```python
from build123d import *

# Parameters (mm, degrees)
SKETCH3_R               = 28
BOSS_EXTRUDE1_DEPTH     = 5.15
SKETCH6_R               = 25
BOSS_EXTRUDE4_DEPTH     = 7
SKETCH7_R               = 3.4
BOSS_EXTRUDE5_DEPTH     = 10
CUT_EXTRUDE1_DEPTH      = 10
CUT_EXTRUDE1_DEPTH_BACK = 43.3971992
SKETCH8_R               = 1.65
CUT_EXTRUDE3_DEPTH      = 2.7
CHAMFER1_SIZE           = 1


with BuildPart() as part:
    # Sketch3 → Boss-Extrude1 (new body)
    with BuildSketch(Plane(origin=(0, 0, 0), x_dir=(1, 0, 0), z_dir=(0, 1, 0))):
        with Locations(Location((0, 0, 0), (0, 0, 90))):
            Circle(SKETCH3_R)
    extrude(amount=BOSS_EXTRUDE1_DEPTH)

    # Sketch6 → Boss-Extrude4 (add)
    with BuildSketch(Plane.XZ):
        with Locations(Location((0, 0, 0), (0, 0, 270))):
            Circle(SKETCH6_R)
    extrude(amount=BOSS_EXTRUDE4_DEPTH)

    # Sketch7 → Boss-Extrude5 (add)
    with BuildSketch(Plane(origin=(0, 5.15, 0), x_dir=(1, 0, 0), z_dir=(0, 1, 0))):
        with Locations(Location((-0.954174099, -21.854179847, 0), (0, 0, 270))):
            Circle(SKETCH7_R)
        with Locations(Location((-18.449187877, 11.753428933, 0), (0, 0, 270))):
            Circle(SKETCH7_R)
        with Locations(Location((19.403361976, 10.100750915, 0), (0, 0, 270))):
            Circle(SKETCH7_R)
    extrude(amount=BOSS_EXTRUDE5_DEPTH)

    # Sketch8 → Cut-Extrude1 (cut, two sides: drawn at the far end of the back side and taken through both)
    with BuildSketch(Plane.XZ.offset(-CUT_EXTRUDE1_DEPTH_BACK)):
        with Locations(Location((20, 0, 0), (0, 0, 90))):
            Circle(SKETCH8_R)
        with Locations(Location((-20, 0, 0), (0, 0, 90))):
            Circle(SKETCH8_R)
        with Locations(Location((11.471528727, 16.383040886, 0), (0, 0, 90))):
            Circle(SKETCH8_R)
        with Locations(Location((-11.471528727, -16.383040886, 0), (0, 0, 90))):
            Circle(SKETCH8_R)
        with Locations(Location((11.471528727, -16.383040886, 0), (0, 0, 90))):
            Circle(SKETCH8_R)
        with Locations(Location((-11.471528727, 16.383040886, 0), (0, 0, 90))):
            Circle(SKETCH8_R)
    extrude(amount=CUT_EXTRUDE1_DEPTH + CUT_EXTRUDE1_DEPTH_BACK, mode=Mode.SUBTRACT)

    # Sketch11 → Cut-Extrude3 (cut)
    with BuildSketch(Plane(origin=(0, 5.15, 0), x_dir=(1, 0, 0), z_dir=(0, 1, 0))):
        Polygon((11.858091258, -19.360271603), (14.243167426, -17.536883273), (13.856604896, -14.559652555), (11.084966196, -13.405810169), (8.699890028, -15.229198499), (9.086452558, -18.206429216), align=None)
        Polygon((-12.091418901, -19.320568674), (-9.237500125, -18.388645418), (-8.617609951, -15.45111763), (-10.851638553, -13.445513098), (-13.705557329, -14.377436353), (-14.325447503, -17.314964141), align=None)
        Polygon((-22.590586111, -1.517299224), (-19.981273382, -3.002162995), (-17.390687271, -1.48486377), (-17.409413889, 1.517299224), (-20.018726618, 3.002162995), (-22.609312729, 1.48486377), align=None)
        Polygon((20, -3.0022214), (22.6, -1.5011107), (22.6, 1.5011107), (20, 3.0022214), (17.4, 1.5011107), (17.4, -1.5011107), align=None)
        Polygon((9.008253879, 14.666762832), (11.726231698, 13.391643264), (14.189506546, 15.107921318), (13.934803575, 18.09931894), (11.216825756, 19.374438507), (8.753550908, 17.658160453), align=None)
        Polygon((-10.729703857, 13.473912288), (-8.581237024, 15.57091577), (-9.323061894, 18.480044367), (-12.213353597, 19.292169483), (-14.36182043, 17.195166002), (-13.61999556, 14.286037405), align=None)
    extrude(amount=-CUT_EXTRUDE3_DEPTH, mode=Mode.SUBTRACT)

    # Chamfer1
    chamfer1_edges = [part.edges().sort_by_distance(p)[0] for p in [
        (-18.449187877, 5.15, -15.153428933),
        (-0.954174099, 5.15, 18.454179847),
        (19.403361976, 5.15, -13.500750915),
    ]]
    chamfer(chamfer1_edges, length=CHAMFER1_SIZE)


solid = part.part
```
Design review of the part built by this model. Coordinates are the model's own, in mm. A direction names the side the tool comes from. Give positions to 0.01 mm unless a question says otherwise; leave off trailing zeros. Loops run counter-clockwise (first coordinate to the right, second up) from the corner with the lowest first, then second, coordinate; pieces in that order, holes last. Notation, with made-up numbers: M 9.5,69 L 35.5,69 A24 cw 35.5,96 Z; hole C 28,47.5 d9. An arc over 180 degrees is marked long. Return JSON: item names as keys, results as strings. Group by question number.
Item 1: For probe 1 along X at (y, z) = (1.75, 17); probe 2 along X at (y, z) = (-0.5, -0.5) (3 decimals); probe 3 along Y at (x, z) = (15, 10), list the stretches that pass through material, from the lowest coordinate up.
Item 2: We need section B-B (y = -0.75). Give the boundary of the cut face in (x, z), and give its area (3 significant figures).
Item 3: We need section C-C (y = 7.75). Give the boundary of the cut face in (x, z).
Item 4: Insertion check: pin 1 Ø4.5 at (x, z) = (11.5, 15.5) entering from +Y; pin 2 Ø12 at (x, y) = (-20, -2.5) entering from -Z; pin 3 Ø4 at (x, z) = (11.47, 16.38) entering from +Y; pin 4 Ø2.5 at (x, z) = (11.47, -16.38) entering from -Y. Each pin has a flat end and moves straight along its axis. Give the tip position at first contact, or say it passes through.
Item 5: We need section A-A (z = 16.5). Give the boundary of the cut face in (x, y), and give its area (3 significant figures).
Item 6: Mouldability with a two-part tool opening along X and no side actions: class faces 3 (the flat face through (-10, 2.45, 18)), 4 (the flat face through (-1, 15.15, 22)) as released by +X, released by -X, zero draft, split by the parting line, or undercut.
Item 7: Tool access review of faces 1 (the flat face through (-12.259, 3.819, 13.905)), 2 (the cylindrical face through (12.103, -2.209, -14.859)): name each direction out of +Z, -Z, +X, -X, +Y, -Y from which nothing blocks a thin tool from reaching the whole face with its end or side.
Item 8: We need section D-D (z = -23). Give the boundary of the cut face in (x, y).
Output:
{
 "1": {"probe 1": "x = -22.25 to -13, -9.94 to 9.94, 13 to 22.25", "probe 2": "x = -24.995 to -21.572, -18.428 to 18.428, 21.572 to 24.995", "probe 3": "y = -7 to 5.15"},
 "2": {"outline": "C 0,0 d50; hole C -20,0 d3.3; hole C -11.47,-16.38 d3.3; hole C -11.47,16.38 d3.3; hole C 11.47,-16.38 d3.3; hole C 11.47,16.38 d3.3; hole C 20,0 d3.3", "area": "1,910 mm^2"},
 "3": {"outline": "C -18.45,-11.75 d6.8; C -0.95,21.85 d6.8; C 19.4,-10.1 d6.8"},
 "4": {"pin 1": "stops at y = 5.15", "pin 2": "stops at z = -23.93", "pin 3": "stops at y = 2.45", "pin 4": "passes through"},
 "5": {"outline": "M -22.62,0 L -18.78,0 L -18.78,-7 L -13.12,-7 L -13.12,2.45 L -14.15,2.45 L -14.15,5.15 L -22.62,5.15 Z; M -9.83,-7 L 9.83,-7 L 9.83,2.45 L 8.86,2.45 L 8.86,5.15 L -8.84,5.15 L -8.84,2.45 L -9.83,2.45 Z; M 13.12,-7 L 18.78,-7 L 18.78,0 L 22.62,0 L 22.62,5.15 L 14.11,5.15 L 14.11,2.45 L 13.12,2.45 Z", "area": "405 mm^2"},
 "6": {"face 3": "undercut", "face 4": "zero draft"},
 "7": {"face 1": "+Y", "face 2": "+Y, -Y"},
 "8": {"outline": "M -15.97,0 L -9.8,0 L -9.8,-7 L 9.8,-7 L 9.8,0 L 15.97,0 L 15.97,5.15 L -15.97,5.15 Z"}
}
